Read the model definition and answer for the solid it produces. Units are mm, in the model's axes. A direction names the side the tool comes from. Round coordinates to 2 decimals unless told otherwise and drop trailing zeros. Loops run counter-clockwise (first coordinate to the right, second up) from the corner with the lowest first, then second, coordinate; pieces in that order, holes last. Notation, with made-up numbers: (1.25, 57.5) -> (10.25, 57.5) arc R15 cw to (10.25, 85.5) -> close; hole circle Ø11 at (34.25, -16.75). An arc over 180 degrees is marked (long way). Put each result on its own line as item: value.
from build123d import *

# Parameters (mm, degrees)
F1_DEPTH = 1.8
F2_DEPTH = 1.2
F4_DEPTH = 1.2
F5_R     = 1
F6_R     = 0.5
F7_DEPTH = 12.5
F8_R     = 0.5
F9_DEPTH = 1.2


with BuildPart() as f1:
    # F0 (on Front) → F1 (new body)
    with BuildSketch(Plane.XZ):
        with BuildLine():
            Line((5, 0), (0, 5))
            Line((0, 5), (-1.249147, 3.750853))
            ThreePointArc((-1.249147, 3.750853), (-0.864917, 0), (-1.249147, -3.750853))
            Line((-1.249147, -3.750853), (0, -5))
            Line((0, -5), (5, 0))
        make_face()
    extrude(amount=F1_DEPTH)

    # F0 (on Front) → F2 (join)
    with BuildSketch(Plane.XZ):
        with BuildLine():
            ThreePointArc((-1.249147, -3.750853), (-0.864917, 0), (-1.249147, 3.750853))
            Line((-1.249147, 3.750853), (-5, 0))
            Line((-5, 0), (-1.249147, -3.750853))
        make_face()
    extrude(amount=F2_DEPTH)

    # F3 (on face) → F4 (cut)
    with BuildSketch(Plane.XZ):
        with BuildLine():
            ThreePointArc((1.249147, 3.750853), (0.864917, 0), (1.249147, -3.750853))
            Line((1.249147, -3.750853), (5, 0))
            Line((5, 0), (1.249147, 3.750853))
        make_face()
    extrude(amount=F4_DEPTH, mode=Mode.SUBTRACT)

    # F5
    f5_edges = [f1.edges().sort_by_distance(p)[0] for p in [
        (0, -0.9, 5),
        (5, -1.5, 0),
        (0, -0.9, -5),
        (-5, -0.6, 0),
    ]]
    fillet(f5_edges, radius=F5_R)

    # F6 (on Front) → F7 (cut, symmetric)
    with BuildSketch(Plane.XZ):
        with Locations((-2.72579, 0)):
            Circle(F6_R)
        with Locations((0, 3)):
            Circle(F6_R)
        with Locations((0, -3)):
            Circle(F6_R)
    extrude(amount=F7_DEPTH, both=True, mode=Mode.SUBTRACT)

    # F8 (on face) → F9 (join)
    with BuildSketch(Plane(origin=(0, -1.2, 0), x_dir=(-1, 0, 0), z_dir=(0, 1, 0))):
        with Locations((-2.72579, 0)):
            Circle(F8_R)
    extrude(amount=F9_DEPTH)


solid = f1.part
Item 1: The part is cut by section A-A (y = -0.9). Determine the outline of the cut face in (x, z), then the cut area to 3 significant figures.
Derived:
outline: (-4.29, -0.71) -> (-0.71, -4.29) arc R1 ccw to (0.71, -4.29) -> (1.25, -3.75) arc R18.5 cw to (1.25, 3.75) -> (0.71, 4.29) arc R1 ccw to (-0.71, 4.29) -> (-4.29, 0.71) arc R1 ccw to start; circle Ø1 at (2.73, 0); hole circle Ø1 at (-2.73, 0); hole circle Ø1 at (0, -3); hole circle Ø1 at (0, 3)
area: 31.8 mm^2
Item 2: For a pull along Z with two mould halves and no side action, classify faces 3 (the flat face through (-2, -1.2, 0)), 4 (the cylindrical face through (-4.586, -0.608, 0.011)), 5 (the cylindrical face through (-3.123, -0.592, -0.304)), 6 (the flat face through (-1, 0, 0)) as pulls with the +Z half, pulls with the -Z half, needs draft (parallel to the pull), parting line crosses it, or undercut.
Derived:
face 3: undercut
face 4: parting line crosses it
face 5: undercut
face 6: needs draft
Item 3: Flat-ended cylindrical pins translate along their axes: pin 1 Ø1 at (y, z) = (-1.5, 1.5) entering from -X; pin 2 Ø4 at (x, z) = (-3.5, 1) entering from -Y. Find the tip coordinate at first contact, or state that the pin passes through.
Derived:
pin 1: stops at x = -3.9
pin 2: stops at y = -1.2
Item 4: The part is cut by section B-B (x = 0). Determine the outline of the cut face in (y, z), then the cut area to 3 significant figures.
Derived:
outline: (-1.8, -4.59) -> (0, -4.59) -> (0, -3.5) -> (-1.8, -3.5) -> close; (-1.8, -2.5) -> (0, -2.5) -> (0, 2.5) -> (-1.8, 2.5) -> close; (-1.8, 3.5) -> (0, 3.5) -> (0, 4.59) -> (-1.8, 4.59) -> close
area: 12.9 mm^2
Item 5: The part is cut by section C-C (z = 3). Determine the outline of the cut face in (x, y).
Derived:
outline: (-2, -1.2) -> (-1.11, -1.2) -> (-1.11, -1.8) -> (-0.5, -1.8) -> (-0.5, 0) -> (-2, 0) -> close; (0.5, -1.8) -> (2, -1.8) -> (2, -1.2) -> (1.11, -1.2) -> (1.11, 0) -> (0.5, 0) -> close
Item 6: The part is cut by section D-D (y = -1.6). Determine the outline of the cut face in (x, z), then the cut area to 3 significant figures.
Derived:
outline: (-1.25, -3.75) -> (-0.71, -4.29) arc R1 ccw to (0.71, -4.29) -> (4.29, -0.71) arc R1 ccw to (4.29, 0.71) -> (0.71, 4.29) arc R1 ccw to (-0.71, 4.29) -> (-1.25, 3.75) arc R18.5 cw to start; hole circle Ø1 at (0, -3); hole circle Ø1 at (0, 3)
area: 31.8 mm^2
Item 7: Find the intervals of material crossed by line 1 along Z through (x, y) = (0, -1.4); line 2 along Z through (x, y) = (-3.75, -0.95); line 3 along Y through (x, z) = (-2.25, 2.5), in increasing order.
Derived:
line 1: z = -4.59 to -3.5, -2.5 to 2.5, 3.5 to 4.59
line 2: z = -1.25 to 1.25
line 3: y = -1.2 to 0
Item 8: Which of the six approach directions +Z, -Z, +X, -X, +Y, -Y give full straight-line access (tool end or side, diameter ignored) to faces 1 (the cylindrical face through (3.123, -0.608, -0.304)), 2 (the cylindrical face through (-0.065, -0.887, 3.496))?
Derived:
face 1: +Y
face 2: +Y, -Y
